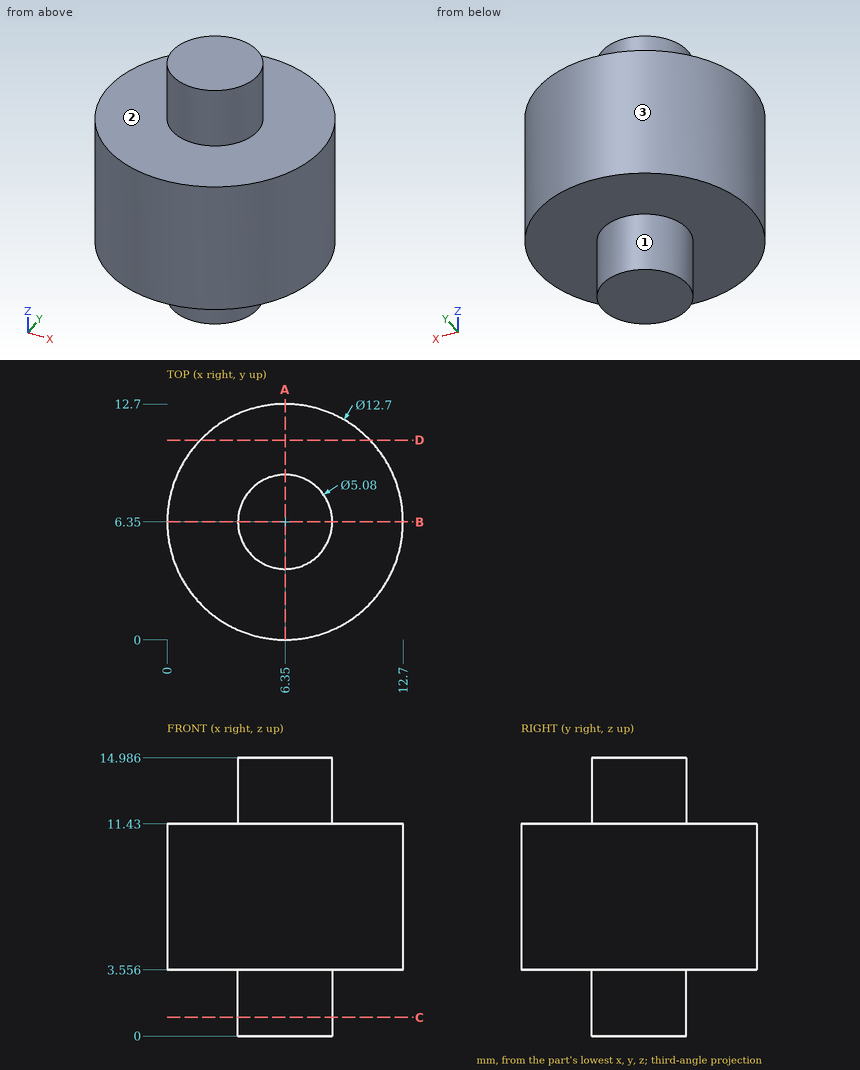
Design review of the part shown in the three views and the two pictorial views. Dimensions are in mm from the part's minimum x, y and z. A direction names the side the tool comes from. Coordinates: 2 decimals unless noted, no trailing zeros. Write each loop counter-clockwise with the first axis right and the second up, starting at its lowest first coordinate (ties: lowest second). Pieces come first, ordered by that corner, then holes. Notation, with made-up numbers: (-21, 55.5) - (-12, 55.5) arc R21 ccw to (-12, 92.5) - close; hole circle Ø4 at (64, 17.5). An arc over 180 degrees is marked (long way). Write item = value, one per line.
(1) Consider section D-D, the plane y = 10.75. Give the boundary of the cut face in (x, z).
Result sheet:
outline = (1.77, 3.56) - (10.93, 3.56) - (10.93, 11.43) - (1.77, 11.43) - close
(2) For line 1 (Z direction, x = 6.25, y = 9); line 2 (X direction, y = 6.25, z = 13.25); line 3 (X direction, y = 6.5, z = 5.5), list the stretches that pass through material, from the lowest coordinate up. Write a range as [from, to].
Result sheet:
line_1 = [3.56, 11.43]
line_2 = [3.81, 8.89]
line_3 = [0, 12.7]
(3) Consider section C-C, the plane z = 1. Give the boundary of the cut face in (x, y), then the cut area to 3 significant figures.
Result sheet:
outline = circle Ø5.08 at (6.35, 6.35)
area = 20.3 mm^2
(4) Consider section A-A, the plane x = 6.35. Give the boundary of the cut face in (y, z), then the cut area to 3 significant figures.
Result sheet:
outline = (0, 3.56) - (3.81, 3.56) - (3.81, 0) - (8.89, 0) - (8.89, 3.56) - (12.7, 3.56) - (12.7, 11.43) - (8.89, 11.43) - (8.89, 14.99) - (3.81, 14.99) - (3.81, 11.43) - (0, 11.43) - close
area = 136 mm^2
(5) For P1, Ø1, axis at x = 7.5, z = 8, coming from the +Y side; P2, Ø1, axis at y = 10.5, z = 6.5, coming from the -X side; P3, Ø2, axis at y = 4.5, z = 13.5, coming from the +X side, all flat-tipped, find the tip position at first contact; note any pin that passes through.
Result sheet:
P1 = 12.67
P2 = 1.15
P3 = 8.74
(6) Machinability: for the marked faces 1, 2 and 3, which of the approach directions +Z, -Z, +X, -X, +Y, -Y give a long, thin tool a straight path to every point of the face, cutting with its end or side? Answer none if there is none.
Result sheet:
face_1 = -Z
face_2 = +Z
face_3 = +Z, -Z
